from build123d import *

# Parameters (mm, degrees)
F2_R     = 1.8288
F3_DEPTH = 3.175
F4_R     = 1.8288
F4_R_2   = 6.35
F5_DEPTH = 22.2550495781


with BuildPart() as f1:
    # F0 (on Top) → F1 (revolve)
    with BuildSketch(Plane.XY):
        with BuildLine():
            ThreePointArc((-36.4561261994, 17.1794718059), (-16.929171458, 11.3460812753), (0, 0))
            ThreePointArc((0, 0), (2.2342838703, -1.3864951183), (4.8188738006, -1.8705281941))
            Line((4.8188738006, -1.8705281941), (39.7438738006, -1.8705281941))
            Line((39.7438738006, -1.8705281941), (39.7438738006, 1.3044718059))
            Line((39.7438738006, 1.3044718059), (4.8188738006, 1.3044718059))
            ThreePointArc((4.8188738006, 1.3044718059), (3.3831947568, 1.5733408189), (2.1421025074, 2.3435063149))
            ThreePointArc((2.1421025074, 2.3435063149), (-15.7784918037, 14.3133175148), (-36.4561261994, 20.3845213841))
            Line((-36.4561261994, 20.3845213841), (-45.9811261994, 20.3845213841))
            Line((-45.9811261994, 20.3845213841), (-45.9811261994, 17.1794718059))
            Line((-45.9811261994, 17.1794718059), (-36.4561261994, 17.1794718059))
        make_face()
    revolve(axis=Axis((-45.9811261994, 7.6544718059, 0), (0, 1, 0)))

    # F2 (on face) → F3 (cut, through all)
    with BuildSketch(Plane.XZ.offset(1.8705281941)):
        with Locations((-87.2561261994, 71.4903970824)):
            Circle(F2_R)
        with Locations((-4.7061261994, 71.4903970824)):
            Circle(F2_R)
        with Locations((36.5688738006, 0)):
            Circle(F2_R)
        with Locations((-4.7061261994, -71.4903970824)):
            Circle(F2_R)
        with Locations((-87.2561261994, -71.4903970824)):
            Circle(F2_R)
        with Locations((-128.5311261994, 0)):
            Circle(F2_R)
        with Locations((-117.4715232818, 41.275)):
            Circle(F2_R)
        with Locations((25.509270883, 41.275)):
            Circle(F2_R)
        with Locations((-45.9811261994, -82.55)):
            Circle(F2_R)
    extrude(amount=-F3_DEPTH, mode=Mode.SUBTRACT)

    # F4 (on face) → F5 (cut, through all)
    with BuildSketch(Plane.XZ.offset(1.8705281941)):
        with Locations((-109.2226313107, 36.5125)):
            Circle(F4_R)
        with Locations((17.260378912, 36.5125)):
            Circle(F4_R)
        with Locations((-45.9811261994, -73.025)):
            Circle(F4_R)
        with Locations((-45.9811261994, 0)):
            Circle(F4_R_2)
        with Locations((-45.9811261994, 53.975)):
            Circle(F4_R)
        with Locations((-92.7248473687, -26.9875)):
            Circle(F4_R)
        with Locations((0.7625949699, -26.9875)):
            Circle(F4_R)
    extrude(amount=-F5_DEPTH, mode=Mode.SUBTRACT)


solid = f1.part
Design review of the part built by this model. Coordinates are the model's own, in mm. A direction names the side the tool comes from. Coordinates: 2 decimals unless noted, no trailing zeros. Loops run counter-clockwise (first coordinate to the right, second up) from the corner with the lowest first, then second, coordinate; pieces in that order, holes last. Notation, with made-up numbers: (-6, 71.25) -> (1, 71.25) arc R22 ccw to (1, 107.25) -> close; hole circle Ø5 at (36.25, 44.5). An arc over 180 degrees is marked (long way). Use a Markdown table: item, result. Add a question column.
Item 1: We need section B-B, the plane z = 64. Write out the cut boundary in (x, y), and give its area (3 significant figures).
Item 2: Wall thickness on L1, parallel to Y at x = -103.5, z = 46.5; L2, parallel to Z at x = -53.5, y = 3.5; L3, parallel to X at y = 4.5, z = 32.5: over which ranges is each line inside the solid? List them lowest first. Write a range as from..to.
Item 3: We need section A-A, the plane y = 10.5. Write out the cut boundary in (x, z), and give its area (3 significant figures).
Item 4: Clearance check with flat-ended pins moving along their axes: P1, Ø6, axis at x = -45.98, z = 53.98, coming from the -Y side; P2, Ø21, axis at x = -44.5, z = -1.5, coming from the -Y side; P3, Ø6, axis at x = -20, z = 7.5, coming from the -Y side; P4, Ø4, axis at x = 36.57, z = 0, coming from the +Y side. State where each tip first meets the part, or that it passes through.
Item 5: Machinability: for faces 4 (the flat face through (-48, 17.179, 6.2)), 5 (the cylindrical face through (35.118, -0.305, -1.113)), which of the approach directions +Z, -Z, +X, -X, +Y, -Y give a long, thin tool a straight path to every point of the face, cutting with its end or side? Answer none if there is none.
Item 6: The part is to be moulded in two halves that separate along X. For faces 1 (the cylindrical face through (0.104, -0.261, -72.284)), 2 (the flat face through (-9, 1.304, 37)), 3 (the cylindrical face through (-85.567, -0.305, -72.191)), say which applies: +X half, -X half, draft (parallel to the pull), parting line (faces both ways), or undercut.
Numbers:
| question | item | result |
|---|---|---|
| 1 | outline | (-103.01, -1.87) -> (11.05, -1.87) -> (11.05, 1.3) -> (-103.01, 1.3) -> close |
| 1 | area | 362 mm^2 |
| 2 | L1 | y = -1.87..1.3 |
| 2 | L2 | z = -46.22..-41.15, 41.15..46.22 |
| 2 | L3 | x = -78.04..-70.17, -21.79..-13.92 |
| 3 | outline | circle Ø74.58 at (-45.98, 0); hole circle Ø61.57 at (-45.98, 0) |
| 3 | area | 1,390 mm^2 |
| 4 | P1 | stops at y = -1.87 |
| 4 | P2 | stops at y = 16.67 |
| 4 | P3 | stops at y = 10.87 |
| 4 | P4 | stops at y = 1.3 |
| 5 | face 4 | -Y |
| 5 | face 5 | +Y, -Y |
| 6 | face 1 | parting line |
| 6 | face 2 | draft |
| 6 | face 3 | undercut |
